The listing builds one solid part. Answer for the finished solid, in the listing's coordinates (mm). A direction names the side the tool comes from. Coordinates: 2 decimals unless noted, no trailing zeros. Order: outer loops, then holes, each group sorted by start corner. A loop starts at its lowest first (then second) coordinate and runs counter-clockwise, first axis right, second up. Notation, with made-up numbers: (26, 7) -> (74, 7) arc R22 ccw to (74, 27) -> close; hole circle Ø6 at (-26.5, 21). An arc over 180 degrees is marked (long way). Return JSON: item names as keys, results as strings.
```python
from build123d import *

# Parameters (mm, degrees)
SKETCH1_R           = 1.75
SKETCH1_W           = 20.2
SKETCH1_H           = 20.2
BOSS_EXTRUDE1_DEPTH = 4.7625
FILLET1_R           = 6
FILLET2_R           = 10
SKETCH2_W           = 6.35
SKETCH2_H           = 20.2
BOSS_EXTRUDE2_DEPTH = 19.05
SKETCH3_R           = 2.286
CUT_EXTRUDE1_DEPTH  = 57.45
SKETCH4_W           = 32.9
SKETCH4_H           = 6.35
BOSS_EXTRUDE3_DEPTH = 12
FILLET5_R           = 6.35


with BuildPart() as part:
    # Sketch1 → Boss-Extrude1 (new body)
    with BuildSketch(Plane.XY):
        Polygon((-30, -30), (0, -16.45), (17, -36), (27, -36), (27, -26), (16.45, 0), (27, 26), (27, 36), (17, 36), (0, 16.45), (-30, 30), (-40, 30), (-40, 20), (-16.45, 0), (-40, -20), (-40, -30), align=None)
        with Locations((22, 31)):
            Circle(SKETCH1_R, mode=Mode.SUBTRACT)
        with Locations((22, -31)):
            Circle(SKETCH1_R, mode=Mode.SUBTRACT)
        with Locations((-35, 25)):
            Circle(SKETCH1_R, mode=Mode.SUBTRACT)
        with Locations((-35, -25)):
            Circle(SKETCH1_R, mode=Mode.SUBTRACT)
        Rectangle(SKETCH1_W, SKETCH1_H, mode=Mode.SUBTRACT)
    extrude(amount=BOSS_EXTRUDE1_DEPTH)

    # Fillet1
    fillet1_edges = [part.edges().sort_by_distance(p)[0] for p in [
        (17, 36, 2.38125),
        (27, 36, 2.38125),
        (27, 26, 2.38125),
        (27, -26, 2.38125),
        (27, -36, 2.38125),
        (17, -36, 2.38125),
        (-30, -30, 2.38125),
        (-40, -30, 2.38125),
        (-40, -20, 2.38125),
        (-40, 20, 2.38125),
        (-40, 30, 2.38125),
        (-30, 30, 2.38125),
    ]]
    fillet(fillet1_edges, radius=FILLET1_R)

    # Fillet2
    fillet2_edges = [part.edges().sort_by_distance(p)[0] for p in [
        (0, 16.45, 2.38125),
        (16.45, 0, 2.38125),
        (0, -16.45, 2.38125),
        (-16.45, 0, 2.38125),
    ]]
    fillet(fillet2_edges, radius=FILLET2_R)

    # Sketch2 → Boss-Extrude2 (add)
    with BuildSketch(Plane.XY.offset(4.7625)):
        with Locations((13.275, 0)):
            Rectangle(SKETCH2_W, SKETCH2_H)
        with Locations((-13.275, 0)):
            Rectangle(SKETCH2_W, SKETCH2_H)
    extrude(amount=BOSS_EXTRUDE2_DEPTH)

    # Sketch3 → Cut-Extrude1 (cut, through all)
    with BuildSketch(Plane(origin=(16.45, 0, 0), x_dir=(0, 0, -1), z_dir=(1, 0, 0))):
        with Locations((-14.2875, 0)):
            Circle(SKETCH3_R)
    extrude(amount=-CUT_EXTRUDE1_DEPTH, mode=Mode.SUBTRACT)

    # Sketch4 → Boss-Extrude3 (add)
    with BuildSketch(Plane.XY.offset(4.7625)):
        with Locations((0, 13.275)):
            Rectangle(SKETCH4_W, SKETCH4_H)
        with Locations((0, -13.275)):
            Rectangle(SKETCH4_W, SKETCH4_H)
    extrude(amount=BOSS_EXTRUDE3_DEPTH)

    # Fillet5
    fillet5_edges = [part.edges().sort_by_distance(p)[0] for p in [
        (13.275, -10.1, 23.8125),
        (13.275, 10.1, 23.8125),
        (-13.275, 10.1, 23.8125),
        (-13.275, -10.1, 23.8125),
    ]]
    fillet(fillet5_edges, radius=FILLET5_R)


solid = part.part
```
Item 1: The part is cut by section C-C on z = 10. Determine the outline of the cut face in (x, y), plus the area to 3 significant figures.
Answer list:
{"outline": "(-16.45, -16.45) -> (16.45, -16.45) -> (16.45, 16.45) -> (-16.45, 16.45) -> close; hole (-10.1, -10.1) -> (10.1, -10.1) -> (10.1, 10.1) -> (-10.1, 10.1) -> close", "area": "674 mm2"}
Item 2: Flat-ended cylindrical pins translate along their axes: pin 1 (5 mm diameter, centred on y = -20, z = 18.5, fed in from -X); pin 2 (3 mm diameter, centred on x = -33, z = 3.5, fed in from +Y); pin 3 (1.9 mm diameter, centred on x = 1.5, y = -12, fed in from +Z); pin 4 (10 mm diameter, centred on x = -14.5, z = 20, fed in from +Y). Find the tip coordinate at first contact, or state that the pin passes through.
Answer list:
{"pin 1": "through", "pin 2": "y = 30", "pin 3": "z = 16.76", "pin 4": "y = 16.45"}
Item 3: Determine the mould class of faces 1 (the cylindrical face through (-13.23, -8.19, 22)), 2 (the cylindrical face through (20.25, 31.08, 2.35)), 3 (the flat face through (-14, 1, 0)), 4 (the cylindrical face through (-13.23, 8.29, 21.9)) for opening direction Y: pulls with the +Y half, pulls with the -Y half, needs draft (parallel to the pull), parting line crosses it, or undercut.
Answer list:
{"face 1": "pulls with the -Y half", "face 2": "undercut", "face 3": "needs draft", "face 4": "pulls with the +Y half"}
Item 4: Find the intervals of material crossed by probe 1 along X at (y, z) = (2, 6.75); probe 2 along Y at (x, z) = (-35, 2); probe 3 along Y at (x, z) = (23, 3.5), in increasing order.
Answer list:
{"probe 1": "-16.45 to -10.1, 10.1 to 16.45", "probe 2": "-29.92 to -26.75, -23.25 to -15.75, 15.75 to 23.25, 26.75 to 29.92", "probe 3": "-35.66 to -32.44, -29.56 to -16.14, 16.14 to 29.56, 32.44 to 35.66"}
Item 5: The part is cut by section B-B on x = 0. Determine the outline of the cut face in (y, z), plus the area to 3 significant figures.
Answer list:
{"outline": "(-18.99, 0) -> (-10.1, 0) -> (-10.1, 16.76) -> (-16.45, 16.76) -> (-16.45, 4.76) -> (-18.99, 4.76) -> close; (10.1, 0) -> (18.99, 0) -> (18.99, 4.76) -> (16.45, 4.76) -> (16.45, 16.76) -> (10.1, 16.76) -> close", "area": "237 mm2"}
Item 6: The part is cut by section A-A on y = 0. Determine the outline of the cut face in (x, z), plus the area to 3 significant figures.
Answer list:
{"outline": "(-21.9, 0) -> (-10.1, 0) -> (-10.1, 12) -> (-16.45, 12) -> (-16.45, 4.76) -> (-21.9, 4.76) -> close; (-16.45, 16.57) -> (-10.1, 16.57) -> (-10.1, 23.81) -> (-16.45, 23.81) -> close; (10.1, 0) -> (17.24, 0) -> (17.24, 4.76) -> (16.45, 4.76) -> (16.45, 12) -> (10.1, 12) -> close; (10.1, 16.57) -> (16.45, 16.57) -> (16.45, 23.81) -> (10.1, 23.81) -> close", "area": "274 mm2"}
Item 7: The part is cut by section D-D on x = 22. Determine the outline of the cut face in (y, z).
Answer list:
{"outline": "(-35.92, 0) -> (-32.75, 0) -> (-32.75, 4.76) -> (-35.92, 4.76) -> close; (-29.25, 0) -> (-13.68, 0) -> (-13.68, 4.76) -> (-29.25, 4.76) -> close; (13.68, 0) -> (29.25, 0) -> (29.25, 4.76) -> (13.68, 4.76) -> close; (32.75, 0) -> (35.92, 0) -> (35.92, 4.76) -> (32.75, 4.76) -> close"}
Item 8: Which of the six approach directions +Z, -Z, +X, -X, +Y, -Y give full straight-line access (tool end or side, diameter ignored) to faces 5 (the cylindrical face through (-39.46, -20.29, 2.41)), 6 (the flat face through (-33, -30, 2)), 7 (the flat face through (0, -13, 16.762)), 8 (the flat face through (22.33, -14.49, 2.35))?
Answer list:
{"face 5": "+Z, -Z, -X", "face 6": "+Z, -Z, -X, -Y", "face 7": "+Z, +X, -X, -Y", "face 8": "+Z, -Z, +X"}
